```python
from build123d import *

# Parameters (mm, degrees)
SKETCH039_W     = 33.930523
SKETCH039_H     = 11
PAD014_DEPTH    = 48
POCKET014_DEPTH = 15
CHAMFER002_SIZE = 2


with BuildPart() as part:
    # Sketch039 (on Face1 of Binder017) → Pad014 (new body)
    with BuildSketch(Plane.XY.offset(25.4)):
        with Locations((70.371465, 14.5)):
            Rectangle(SKETCH039_W, SKETCH039_H)
    extrude(amount=-PAD014_DEPTH)

    # Sketch041 (on Face1 of Binder019) → SubtractiveLoft section 0
    with BuildSketch(Plane(origin=(0, 0, -23.6), x_dir=(1, 0, 0), z_dir=(0, 0, -1))):
        Polygon((56.284717, -14), (84.458214, -14), (81.571463, -9), (59.171468, -9), align=None)
    # Sketch040 (on Face1 of Binder018) → SubtractiveLoft section 1
    with BuildSketch(Plane.XY.offset(-1.6)):
        Polygon((58.406204, 14), (82.336727, 14), (79.449975, 9), (61.292955, 9), align=None)
    loft(mode=Mode.SUBTRACT)

    # SubtractiveLoft Face6 → Pocket014 (cut)
    with BuildSketch(Plane(origin=(70.371465, 11.614315, -1.6), x_dir=(0, -1, 0), z_dir=(0, 0, -1))):
        Polygon((-2.385685, 11.965261), (-2.385685, -11.965261), (2.614315, -9.07851), (2.614315, 9.07851), align=None)
    extrude(amount=-POCKET014_DEPTH, mode=Mode.SUBTRACT)

    # Chamfer002
    chamfer002_edges = [part.edges().sort_by_distance(p)[0] for p in [
        (87.336727, 14.5, 25.4),
        (87.336727, 20, 1.4),
        (70.371465, 20, 25.4),
        (53.406204, 14.5, 25.4),
        (53.406204, 20, 1.4),
        (53.406204, 14.5, -22.6),
        (70.371465, 20, -22.6),
        (87.336727, 14.5, -22.6),
    ]]
    chamfer(chamfer002_edges, length=CHAMFER002_SIZE)


solid = part.part
```
Could you check a few things on this model? Use its own coordinates, in mm. A direction names the side the tool comes from. Round coordinates to 2 decimals unless told otherwise and drop trailing zeros. Loops run counter-clockwise (first coordinate to the right, second up) from the corner with the lowest first, then second, coordinate; pieces in that order, holes last. Notation, with made-up numbers: M -35.5,86 L -17.5,86 A10 ccw -17.5,101 Z; hole C 67,-29.5 d11. An arc over 180 degrees is marked long. Answer as CSV lines item,"result".
1) Imagine slicing it at B-B on x = 66. List the corners of the cut face in (y, z) for me.
From the geometry:
outline,"M 9,13.4 L 14,13.4 L 14,-22.6 L 18,-22.6 L 20,-20.6 L 20,23.4 L 18,25.4 L 9,25.4 Z"
2) Which directions (+Z, -Z, +X, -X, +Y, -Y) give clear straight access to the entire face, cutting with the end or side of a thin tool? Please do faces 1 (the flat face through (54.774, 18.604, -21.364)), 2 (the flat face through (59.87, 11.465, 5.795)).
From the geometry:
face 1,"-Z, -X, +Y"
face 2,"-Z"
3) Imagine slicing it at A-A on z = 6. List the corners of the cut face in (x, y) for me, and give its area (3 significant figures).
From the geometry:
outline,"M 53.41,9 L 61.29,9 L 58.41,14 L 82.34,14 L 79.45,9 L 87.34,9 L 87.34,18 L 85.34,20 L 55.41,20 L 53.41,18 Z"
area,"264 mm^2"
4) If I drill on probe 1 along Z at (x, y) = (68.5, 12.75); probe 2 along X at (y, z) = (12.5, -3); probe 3 along X at (y, z) = (13, -13.5), over which ranges is the centre line in solid material (lowest first)?
From the geometry:
probe 1,"13.4 to 25.4"
probe 2,"53.41 to 59.14, 81.61 to 87.34"
probe 3,"53.41 to 57.84, 82.91 to 87.34"
5) Imagine slicing it at C-C on y = 19. List the corners of the cut face in (x, z) for me.
From the geometry:
outline,"M 54.41,-20.6 L 55.41,-21.6 L 85.34,-21.6 L 86.34,-20.6 L 86.34,23.4 L 85.34,24.4 L 55.41,24.4 L 54.41,23.4 Z"
6) We'd pull the mould along Y, two halves only. Please class faces 3 (the flat face through (86.351, 13.437, -21.586)), 4 (the flat face through (70.2, 19, 24.4)), 5 (the flat face through (80.91, 11.53, 5.8)): released by +Y, released by -Y, zero draft, split by the parting line, or undercut.
From the geometry:
face 3,"zero draft"
face 4,"released by +Y"
face 5,"undercut"
7) For pin 1 Ø1.5 at (x, y) = (75.5, 12) entering from -Z, with a flat end and sliding along its axis, tell me the tip position at first contact or that it passes through.
From the geometry:
pin 1,"z = 13.4"
